Design review of the part built by this model. Coordinates are the model's own, in mm. A direction names the side the tool comes from. Coordinates: 2 decimals unless noted, no trailing zeros. Order: outer loops, then holes, each group sorted by start corner. A loop starts at its lowest first (then second) coordinate and runs counter-clockwise, first axis right, second up. Notation, with made-up numbers: M 37.25,32.5 L 80.25,32.5 A11 cw 80.25,50.5 Z; hole C 81,-28 d3. An arc over 180 degrees is marked long. Answer in a Markdown table with one row per item.
from build123d import *

# Parameters (mm, degrees)
BOSS_EXTRUDE1_DEPTH = 45
FILLET1_R           = 1
FILLET2_R           = 0.5


with BuildPart() as part:
    # Sketch3 → Boss-Extrude1 (new body)
    with BuildSketch(Plane(origin=(0, 0, 0), x_dir=(0, 0, -1), z_dir=(1, 0, 0))):
        Polygon((-3.729267548, 0), (-5.729267548, 0), (-5.729267548, -5), (-18.229267548, -5), (-18.229267548, -14.5), (-13.131696696, -14.5), (-13.131696696, -12.5), (-14.52244663, -12.5), (-16.229267548, -12.5), (-16.229267548, -7), (-3.729267548, -7), align=None)
        Polygon((-18.229267548, 5), (-5.729267548, 5), (-5.729267548, 0), (-3.729267548, 0), (-3.729267548, 7), (-16.229267548, 7), (-16.229267548, 12.5), (-14.52244663, 12.5), (-13.131696696, 12.5), (-13.131696696, 14.5), (-18.229267548, 14.5), align=None)
    extrude(amount=BOSS_EXTRUDE1_DEPTH)

    # Fillet1
    fillet1_edges = [part.edges().sort_by_distance(p)[0] for p in [
        (22.5, -14.5, 18.229267548),
        (22.5, -5, 18.229267548),
        (22.5, 5, 18.229267548),
        (22.5, 14.5, 18.229267548),
        (22.5, 12.5, 16.229267548),
        (22.5, 7, 16.229267548),
        (22.5, 7, 3.729267548),
        (22.5, -7, 3.729267548),
        (22.5, -7, 16.229267548),
        (22.5, -12.5, 16.229267548),
    ]]
    fillet(fillet1_edges, radius=FILLET1_R)

    # Fillet2
    fillet2_edges = [part.edges().sort_by_distance(p)[0] for p in [
        (22.5, -5, 5.729267548),
        (22.5, 5, 5.729267548),
    ]]
    fillet(fillet2_edges, radius=FILLET2_R)


solid = part.part
(1) Add section B-B, the plane x = 34.5. Give the boundary of the cut face in (y, z), and give its area (3 significant figures).
Return value:
| item | result |
|---|---|
| outline | M -14.5,13.13 L -12.5,13.13 L -12.5,15.23 A1 cw -11.5,16.23 L -8,16.23 A1 cw -7,15.23 L -7,4.73 A1 ccw -6,3.73 L 6,3.73 A1 ccw 7,4.73 L 7,15.23 A1 cw 8,16.23 L 11.5,16.23 A1 cw 12.5,15.23 L 12.5,13.13 L 14.5,13.13 L 14.5,17.23 A1 ccw 13.5,18.23 L 6,18.23 A1 ccw 5,17.23 L 5,6.23 A0.5 cw 4.5,5.73 L -4.5,5.73 A0.5 cw -5,6.23 L -5,17.23 A1 ccw -6,18.23 L -13.5,18.23 A1 ccw -14.5,17.23 Z |
| area | 120 mm2 |
(2) Draft analysis for pull direction Y (two halves, no side actions). For faces 4 (the flat face through (22, -5, 12)), 5 (the flat face through (22, 14.5, 15)), 6 (the cylindrical face through (22.815, -6.715, 4.03)), state which applies: pulls with the +Y half, pulls with the -Y half, needs draft (parallel to the pull), parting line crosses it, or undercut.
Return value:
| item | result |
|---|---|
| face 4 | undercut |
| face 5 | pulls with the +Y half |
| face 6 | pulls with the -Y half |
(3) For line 1 along Y through (x, z) = (40, 14.25); line 2 along Y through (x, z) = (4.5, 10); line 3 along Y through (x, z) = (28.5, 16), list the stretches that pass through material, from the lowest coordinate up. Write a range as from..to.
Return value:
| item | result |
|---|---|
| line 1 | y = -14.5..-12.5, -7..-5, 5..7, 12.5..14.5 |
| line 2 | y = -7..-5, 5..7 |
| line 3 | y = -14.5..-12.14, -7.36..-5, 5..7.36, 12.14..14.5 |
(4) Add section A-A, the plane z = 7.5. Give the boundary of the cut face in (x, y), and give its area (3 significant figures).
Return value:
| item | result |
|---|---|
| outline | M 0,-7 L 45,-7 L 45,-5 L 0,-5 Z; M 0,5 L 45,5 L 45,7 L 0,7 Z |
| area | 180 mm2 |
(5) Add section C-C, the plane z = 14.75. Give the boundary of the cut face in (x, y).
Return value:
| item | result |
|---|---|
| outline | M 0,-14.5 L 45,-14.5 L 45,-12.5 L 0,-12.5 Z; M 0,-7 L 45,-7 L 45,-5 L 0,-5 Z; M 0,5 L 45,5 L 45,7 L 0,7 Z; M 0,12.5 L 45,12.5 L 45,14.5 L 0,14.5 Z |
(6) Add section D-D, the plane y = 10. Give the boundary of the cut face in (x, z), and give its area (3 significant figures).
Return value:
| item | result |
|---|---|
| outline | M 0,16.23 L 45,16.23 L 45,18.23 L 0,18.23 Z |
| area | 90.0 mm2 |
(7) Insertion check: pin 1 Ø3 at (x, y) = (34, -4) entering from +Z; pin 2 Ø0.6 at (x, y) = (31.5, 13.5) entering from -Z; pin 3 Ø4 at (x, y) = (22.5, 10) entering from -Z. Each pin has a flat end and moves straight along its axis. Give the tip position at first contact, or say it passes through.
Return value:
| item | result |
|---|---|
| pin 1 | stops at z = 18.1 |
| pin 2 | stops at z = 13.13 |
| pin 3 | stops at z = 16.1 |
(8) For faces 1 (the flat face through (22, -14, 13.132)), 2 (the flat face through (22, 12.5, 14)), 3 (the flat face through (22, 0, 5.729)), list the 3-axis set-ups (+Z, -Z, +X, -X, +Y, -Y) from which the entire face can be reached by the end or side of a thin tool; tool diameter is ignored.
Return value:
| item | result |
|---|---|
| face 1 | -Z, +X, -X, -Y |
| face 2 | -Z, +X, -X |
| face 3 | +Z, +X, -X |
